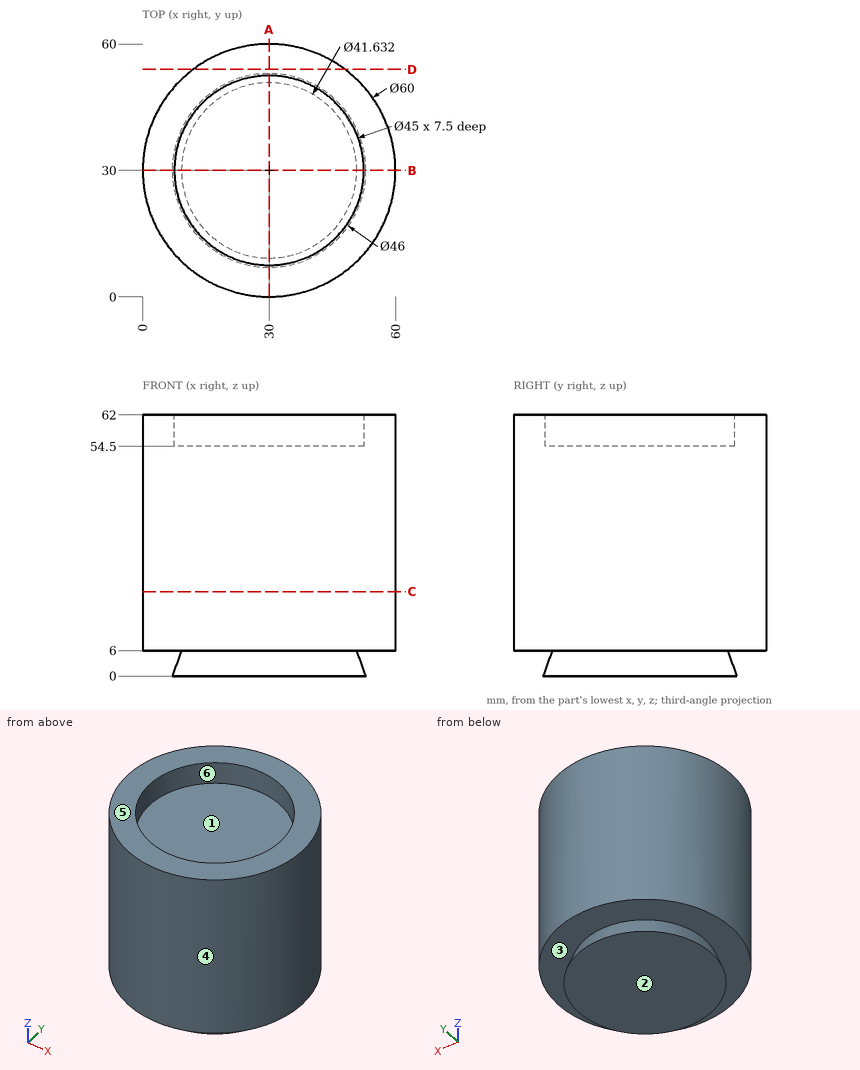
Job drawing, mm, ordinate dimensions from the low corner. One solid piece. A direction names the side the tool comes from. Coordinates: 2 decimals unless noted, no trailing zeros. Order: outer loops, then holes, each group sorted by start corner. A loop starts at its lowest first (then second) coordinate and runs counter-clockwise, first axis right, second up. Notation, with made-up numbers: M 85,77 L 116,77 A16 cw 116,88 Z; hole C -25.75,36 d8. An arc over 180 degrees is marked long. One line per question, with ' | ' between items.
Q1. Drill centre lines: line 1 (Y direction, x = 30, z = 56.25); line 2 (Z direction, x = 32, y = 46); line 3 (X direction, y = 10.5, z = 57.5) (1 decimal). Where is each one in solid material? Low to high.
A:
line 1: y = 0 to 7.5, 52.5 to 60 | line 2: z = 0 to 54.5 | line 3: x = 7.2 to 18.8, 41.2 to 52.8
Q2. Slice it at C-C (z = 20). Give the cut face in (x, y).
A:
outline: C 30,30 d60
Q3. Pin check, flat tips, straight feed: P1, Ø4, axis at x = 34.5, z = 10.5, coming from the +Y side; P2, Ø2, axis at y = 20, z = 34, coming from the +X side; P3, Ø5, axis at x = 15, z = 23, coming from the -Y side. Stop position of each tip, or through.
A:
P1: stops at y = 59.9 | P2: stops at x = 58.62 | P3: stops at y = 2.73
Q4. Slice it at D-D (y = 54). Give the cut face in (x, z), and give its area (3 significant figures).
A:
outline: M 12,6 L 48,6 L 48,62 L 12,62 Z | area: 2,020 mm^2
Q5. Slice it at A-A (x = 30). Give the cut face in (y, z), and give its area (3 significant figures).
A:
outline: M 0,6 L 9.18,6 L 7,0 L 53,0 L 50.82,6 L 60,6 L 60,62 L 52.5,62 L 52.5,54.5 L 7.5,54.5 L 7.5,62 L 0,62 Z | area: 3,290 mm^2
Q6. 3-axis set-ups, long thin cutter, end or side, ignore diameter. For the marked faces 1, 2 and 3: which of +Z, -Z, +X, -X, +Y, -Y reach the whole face in a straight line?
A:
face 1: +Z | face 2: -Z, +X, -X, +Y, -Y | face 3: none
Q7. Two-plate mould, pull along X, no slides. Class the marked faces 4, 5 and 6: +X half, -X half, draft (parallel to the pull), parting line (faces both ways), or undercut.
A:
face 4: parting line | face 5: draft | face 6: undercut
